Build history of the part. All positions in model axes, mm. A direction names the side the tool comes from. Give positions to 0.01 mm unless a question says otherwise; leave off trailing zeros. Write each loop counter-clockwise with the first axis right and the second up, starting at its lowest first coordinate (ties: lowest second). Pieces come first, ordered by that corner, then holes.
from build123d import *

# Parameters (mm, degrees)
F1_R     = 1.6
F1_W     = 20
F1_H     = 5
F1_W_2   = 5
F2_DEPTH = 5


with BuildPart() as f2:
    # F1 (on Right) → F2 (new body)
    with BuildSketch(Plane.YZ):
        with BuildLine():
            Line((0, 5), (0, 0))
            Line((0, 0), (33.5, 0))
            Line((33.5, 0), (33.5, -5))
            Line((33.5, -5), (38.5, -5))
            Line((38.5, -5), (38.5, 0))
            Line((38.5, 0), (47, 0))
            Line((47, 0), (47, 2))
            Line((47, 2), (45.75, 2))
            Line((45.75, 2), (45.75, 5))
            Line((45.75, 5), (47, 5))
            Line((47, 5), (47, 6))
            Line((47, 6), (50, 6))
            Line((50, 6), (50, 5))
            Line((50, 5), (51.25, 5))
            Line((51.25, 5), (51.25, 2))
            Line((51.25, 2), (50, 2))
            Line((50, 2), (50, 0))
            Line((50, 0), (58.5, 0))
            Line((58.5, 0), (58.5, -5))
            Line((58.5, -5), (63.5, -5))
            Line((63.5, -5), (63.5, 0))
            Line((63.5, 0), (97, 0))
            Line((97, 0), (118.2132034356, -21.2132034356))
            Line((118.2132034356, -21.2132034356), (125.2842712475, -28.2842712475))
            Line((125.2842712475, -28.2842712475), (131.2239682094, -34.2239682094))
            Line((131.2239682094, -34.2239682094), (132.9917351624, -32.4562012565))
            Line((132.9917351624, -32.4562012565), (132.178562364, -31.6430284581))
            Line((132.178562364, -31.6430284581), (133.946329317, -29.8752615051))
            Line((133.946329317, -29.8752615051), (135.8908729653, -31.8198051534))
            Line((135.8908729653, -31.8198051534), (137.8354166135, -33.7643488017))
            Line((137.8354166135, -33.7643488017), (136.0676496606, -35.5321157546))
            Line((136.0676496606, -35.5321157546), (135.2544768622, -34.7189429563))
            Line((135.2544768622, -34.7189429563), (133.4867099092, -36.4867099092))
            Line((133.4867099092, -36.4867099092), (139.4264068712, -42.4264068712))
            Line((139.4264068712, -42.4264068712), (146.4974746831, -49.4974746831))
            Line((146.4974746831, -49.4974746831), (153.5685424949, -56.5685424949))
            Line((153.5685424949, -56.5685424949), (179.7314933988, -30.405591591))
            ThreePointArc((179.7314933988, -30.405591591), (180.6101730553, -28.2842712475), (179.7314933988, -26.1629509039))
            Line((179.7314933988, -26.1629509039), (110.8908729653, 42.6776695297))
            ThreePointArc((110.8908729653, 42.6776695297), (102.7802892447, 48.0969883128), (93.2132034356, 50))
            Line((93.2132034356, 50), (0, 50))
            Line((0, 50), (0, 40))
            Line((0, 40), (0, 35))
            Line((0, 35), (5, 35))
            Line((5, 35), (5, 30))
            Line((5, 30), (0, 30))
            Line((0, 30), (0, 10))
            Line((0, 10), (5, 10))
            Line((5, 10), (5, 5))
            Line((5, 5), (0, 5))
        make_face()
        with Locations((2.5, 20)):
            Circle(F1_R, mode=Mode.SUBTRACT)
        with Locations((48.5, 42.5)):
            Rectangle(F1_W, F1_H, mode=Mode.SUBTRACT)
        with Locations((94.5, 7.5)):
            Rectangle(F1_W_2, F1_H, mode=Mode.SUBTRACT)
        with Locations((94.5, 20)):
            Circle(F1_R, mode=Mode.SUBTRACT)
        with Locations((94.5, 32.5)):
            Rectangle(F1_W_2, F1_H, mode=Mode.SUBTRACT)
        Polygon((142.9619407771, -53.033008589), (146.4974746831, -49.4974746831), (139.4264068712, -42.4264068712), (135.8908729653, -45.9619407771), align=None)
        Polygon((125.2842712475, -28.2842712475), (118.2132034356, -21.2132034356), (114.6776695297, -24.7487373415), (121.7487373415, -31.8198051534), align=None)
    extrude(amount=F2_DEPTH)


solid = f2.part
1. Saw through at C-C on y = 87. Give the cut face in (x, z), plus the area to 3 significant figures.
2. Drill centre lines: line 1 along Z through (x, y) = (3.85, 94.5); line 2 along Y through (x, z) = (2, 21); line 3 along Z through (x, y) = (2.25, 56). Where is each one in solid material? Low to high.
3. 3-axis set-ups, long thin cutter, end or side, ignore diameter. For faces 5 (the face through (2.465, 116.47, -22.956)), 6 (the face through (2, 36, -5)), 7 (the face through (2, 94, 35)), 8 (the face through (2, 63.5, -3)): which of +Z, -Z, +X, -X, +Y, -Y reach the whole face in a straight line?
4. Saw through at B-B on y = 161.5. Give the cut face in (x, z), plus the area to 3 significant figures.
5. Mould opens along Z. For faces 1 (the face through (2, 5, 8)), 2 (the face through (2.46, 118.16, -28.23)), 3 (the face through (2, 33.5, -2)), 4 (the face through (2, 94, 5)) say: pulls with the +Z half, pulls with the -Z half, needs draft (parallel to the pull), parting line crosses it, or undercut.
6. Drop flat-ended pins along their axis: pin 1 (1.5 mm diameter, centred on x = 3.5, z = -2.5, fed in from -Y); pin 2 (2.5 mm diameter, centred on x = 1.5, y = 95, fed in from -Z); pin 3 (1.5 mm diameter, centred on x = 3, z = 32.5, fed in from -Y). Give the stop position or say it passes through.
7. Saw through at A-A on x = 0.85. Count the separate pieces of the cut face and the enclosed holes in it, plus the area to 3 significant figures.
Outcome:
1. outline: (0, 0) - (5, 0) - (5, 50) - (0, 50) - close
1. area: 250 mm2
2. line 1: z = 0 to 5, 10 to 18.4, 21.6 to 30, 35 to 49.97
2. line 2: y = 0 to 1.25, 3.75 to 93.25, 95.75 to 132.57
2. line 3: z = 0 to 40, 45 to 50
3. face 5: +X, -X, -Y
3. face 6: -Z, +X, -X, -Y
3. face 7: +X, -X
3. face 8: -Z, +X, -X
4. outline: (0, -48.64) - (5, -48.64) - (5, -7.93) - (0, -7.93) - close
4. area: 204 mm2
5. face 1: undercut
5. face 2: pulls with the -Z half
5. face 3: needs draft
5. face 4: undercut
6. pin 1: stops at y = 33.5
6. pin 2: stops at z = 0
6. pin 3: stops at y = 5
7. separate pieces: 1
7. enclosed holes: 5
7. area: 8,700 mm2
